CAD build for the part. Positions are in the model's coordinates, mm. Face numbers are marked on the shaded views. A direction names the side the tool comes from. Round coordinates to 2 decimals unless told otherwise and drop trailing zeros. Loops run counter-clockwise (first coordinate to the right, second up) from the corner with the lowest first, then second, coordinate; pieces in that order, holes last. Notation, with made-up numbers: M 78,47 L 114,47 A13 cw 114,67 Z; hole C -34.5,27.25 d6. An arc over 180 degrees is marked long. Put each result on its own line as item: value. Start each with the question number.
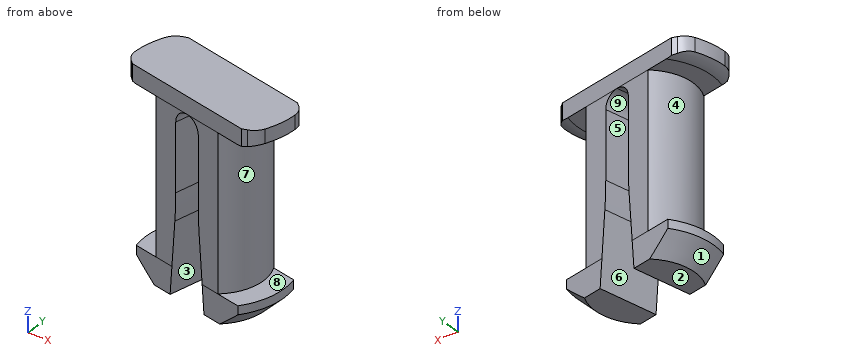
from build123d import *

# Parameters (mm, degrees)
BOSS_EXTRUDE1_DEPTH     = 1
CHAMFER1_SIZE           = 0.5
FILLET1_R               = 1
BOSS_EXTRUDE2_DEPTH     = 8.9
BOSS_EXTRUDE3_DEPTH     = 1.6
CUT_EXTRUDE1_DEPTH      = 63.654658492
CUT_EXTRUDE1_DEPTH_BACK = 63.654658492
FILLET2_R               = 20
FILLET3_R               = 0.8


# Some blends are built 0.0001 mm under size
with BuildPart() as part:
    # Sketch3 → Boss-Extrude1 (new body)
    with BuildSketch(Plane.XY.offset(7.5)):
        with BuildLine():
            Line((-59.471397705, 15.416079883), (-50.967479146, 13.468422533))
            ThreePointArc((-50.967479146, 13.468422533), (-51.028748516, 11.687143573), (-51.748854552, 10.056758353))
            Line((-51.748854552, 10.056758353), (-60.252773111, 12.004415704))
            ThreePointArc((-60.252773111, 12.004415704), (-60.191503741, 13.785694664), (-59.471397705, 15.416079883))
        make_face()
    extrude(amount=-BOSS_EXTRUDE1_DEPTH)

    # Chamfer1
    # the kernel refuses this chamfer: 0.5, 0.404802776 mm, written as the material it takes off along each edge
    with BuildSketch(Plane(origin=(-59.471397705, 15.416079883, 8.793542877), x_dir=(0.9747611941912204, -0.2232501160109568, 0), z_dir=(0, 0, -1))) as chamfer1_piece_1:
        with BuildLine():
            Line((CHAMFER1_SIZE, 0), (-0.128607842, 0.362926907))
            ThreePointArc((-0.128607842, 0.362926907), (-0.070555149, 0.18731274), (0, 0))
            Line((0, 0), (CHAMFER1_SIZE, 0))
        make_face()
    extrude(amount=3.587085755, mode=Mode.SUBTRACT)
    with BuildSketch(Plane(origin=(-50.967479146, 13.468422533, 8.793542877), x_dir=(-0.9747611941912215, 0.22325011601095288, 0), z_dir=(0, 0, -1)), Plane(origin=(-60.252773111, 12.004415704, 8.793542877), x_dir=(0.9747611941912214, -0.22325011601095318, 0), z_dir=(0, 0, -1))) as chamfer1_piece_2:
        with BuildLine():
            Line((CHAMFER1_SIZE, 0), (-0.128607842, -0.362926907))
            ThreePointArc((-0.128607842, -0.362926907), (-0.070555149, -0.18731274), (0, 0))
            Line((0, 0), (CHAMFER1_SIZE, 0))
        make_face()
    extrude(amount=3.587085755, mode=Mode.SUBTRACT)
    with BuildSketch(Plane(origin=(-51.748854552, 10.056758353, 8.793542877), x_dir=(0.5360100963407745, 0.8442115710061985, 0), z_dir=(0, 0, -1))) as chamfer1_piece_3:
        with BuildLine():
            Line((0.385040149, 0), (-CHAMFER1_SIZE * 0.334011510443, -CHAMFER1_SIZE * 0.942568995295))
            Line((-CHAMFER1_SIZE * 0.334011510443, -CHAMFER1_SIZE * 0.942568995295), (0, 0))
            ThreePointArc((0, 0), (0.200121413, 0.003938485), (0.385040149, 0))
        make_face()
    extrude(amount=3.587085755, mode=Mode.SUBTRACT)

    # Fillet1
    fillet1_edges = [part.edges().sort_by_distance(p)[0] for p in [
        (-50.923140687, 13.085943752, 7),
        (-51.542469145, 10.381813703, 7),
        (-59.677783112, 15.091024534, 7),
        (-60.29711157, 12.386894484, 7),
    ]]
    fillet(fillet1_edges, radius=FILLET1_R)

    # Sketch5 → Cut-Revolve1 (revolve, cut)
    with BuildSketch(Plane(origin=(0, 0, 0), x_dir=(0.9747611941912216, -0.22325011601095204, 0), z_dir=(0.22325011601095204, 0.9747611941912216, 0))):
        with BuildLine():
            Line((-60.95, -6.5), (-61.75, -6.5))
            Line((-61.75, -6.5), (-61.75, -6.7))
            ThreePointArc((-61.75, -6.7), (-61.362310563, -6.55075775), (-60.95, -6.5))
        make_face()
    revolve(axis=Axis((-55.610126129, 12.736419118, 6.5), (0, 0, 1)), mode=Mode.SUBTRACT)

    # Sketch6 → Boss-Extrude2 (add)
    with BuildSketch(Plane(origin=(0, 0, 6.5), x_dir=(-1, 0, 0), z_dir=(0, 0, -1))):
        with BuildLine():
            Line((58.131397429, 11.518555813), (56.780622787, 11.209187121))
            Line((56.780622787, 11.209187121), (55.999247381, 14.620851301))
            Line((55.999247381, 14.620851301), (57.350022023, 14.930219993))
            ThreePointArc((57.350022023, 14.930219993), (58.339457472, 13.361519443), (58.131397429, 11.518555813))
        make_face()
        with BuildLine():
            Line((55.221004876, 10.851986936), (53.870230234, 10.542618244))
            ThreePointArc((53.870230234, 10.542618244), (52.880794785, 12.111318794), (53.088854828, 13.954282424))
            Line((53.088854828, 13.954282424), (54.43962947, 14.263651115))
            Line((54.43962947, 14.263651115), (55.221004876, 10.851986936))
        make_face()
    extrude(amount=BOSS_EXTRUDE2_DEPTH)

    # Sketch7 → Boss-Extrude3 (add)
    with BuildSketch(Plane(origin=(0, 0, -2.4), x_dir=(-1, 0, 0), z_dir=(0, 0, -1))):
        with BuildLine():
            Line((54.43962947, 14.263651115), (51.713345578, 13.63924875))
            ThreePointArc((51.713345578, 13.63924875), (51.711081352, 11.843418654), (52.494720985, 10.227584571))
            Line((52.494720985, 10.227584571), (55.221004876, 10.851986936))
            Line((55.221004876, 10.851986936), (54.43962947, 14.263651115))
        make_face()
        with BuildLine():
            Line((55.999247381, 14.620851301), (58.725531273, 15.245253666))
            ThreePointArc((58.725531273, 15.245253666), (59.509170905, 13.629419582), (59.506906679, 11.833589487))
            Line((59.506906679, 11.833589487), (56.780622787, 11.209187121))
            Line((56.780622787, 11.209187121), (55.999247381, 14.620851301))
        make_face()
    extrude(amount=BOSS_EXTRUDE3_DEPTH)

    # Sketch8 → Cut-Revolve2 (revolve, cut)
    with BuildSketch(Plane(origin=(0, 0, 0), x_dir=(0.9747611941912216, -0.22325011601095204, 0), z_dir=(0.22325011601095204, 0.9747611941912216, 0))):
        Polygon((-61.05, 2.9), (-59.95, 4), (-61.05, 4), align=None)
    revolve(axis=Axis((-55.610126129, 12.736419118, 6.5), (0, 0, 1)), mode=Mode.SUBTRACT)

    # Sketch9 → Cut-Extrude1 (cut, two sides: drawn at the far end of the back side and taken through both)
    with BuildSketch(Plane(origin=(0.390687703, 1.70583209, 0), x_dir=(0.9747611941912216, -0.22325011601095204, 0), z_dir=(0.22325011601095204, 0.9747611941912216, 0)).offset(-CUT_EXTRUDE1_DEPTH_BACK)):
        Polygon((-58.25, 4), (-57.85, -1), (-57.85, 4), align=None)
        Polygon((-55.85, 4), (-56.25, -1), (-56.25, 4), align=None)
    extrude(amount=CUT_EXTRUDE1_DEPTH + CUT_EXTRUDE1_DEPTH_BACK, mode=Mode.SUBTRACT)

    # Fillet2
    # the kernel refuses this fillet: 20 mm, written as the material it takes off along each edge
    with BuildSketch(Plane(origin=(-53.993841362, 16.21006421, 1), x_dir=(0, 0, 1), z_dir=(-0.22325011601095204, -0.9747611941912216, 0))) as fillet2_piece_1:
        with BuildLine():
            CenterArc((FILLET2_R * 0.0399362039845, -FILLET2_R), FILLET2_R, 90, 4.57392126)
            Line((-FILLET2_R * 0.0398090182984, -FILLET2_R * 0.00318472146388), (0, 0))
            Line((0, 0), (FILLET2_R * 0.0399362039845, 0))
        make_face()
    extrude(amount=7.493620398, mode=Mode.SUBTRACT)
    with BuildSketch(Plane(origin=(-57.226410896, 9.262774027, 1), x_dir=(-0.07773254810353018, 0.01780313012597799, -0.9968152785361237), z_dir=(0.223250116010952, 0.9747611941912216, 0))) as fillet2_piece_2:
        with BuildLine():
            CenterArc((FILLET2_R * 0.0399362039845, FILLET2_R), FILLET2_R, 265.42607874, 4.57392126)
            Line((-FILLET2_R * 0.0398090182984, FILLET2_R * 0.00318472146388), (0, 0))
            Line((0, 0), (FILLET2_R * 0.0399362039845, 0))
        make_face()
    extrude(amount=7.493620398, mode=Mode.SUBTRACT)

    # Fillet3
    fillet3_edges = [part.edges().sort_by_distance(p)[0] for p in [
        (-54.830317173, 12.557819026, 6.5),
        (-56.389935084, 12.915019211, 6.5),
    ]]
    fillet(fillet3_edges, radius=FILLET3_R - 0.0001)  # a hair under: the kernel refuses the full size


solid = part.part
(1) Flat gauge pins, fed straight in: pin 1 Ø3 at (y, z) = (14, 4) entering from -X; pin 2 Ø5 at (x, z) = (-59, -2.5) entering from -Y; pin 3 Ø4 at (x, z) = (-56, 2.5) entering from -Y. Where does each tip first touch, or does it go through?
(2) Mould opens along X. For the marked faces 6, 7, 8 and 9 say: +X half, -X half, draft (parallel to the pull), parting line (faces both ways), or undercut.
(3) Cut at A-A on z = 3.5. List the corners of the cut face in (x, y).
(4) Drill centre lines: line 1 along Z through (x, y) = (-58.5, 14.85); line 2 along Z through (x, y) = (-52.5, 13.5); line 3 along X through (y, z) = (12.1, 5.75) (3 decimals). Where is each one in solid material? Low to high.
(5) Tool access for the marked faces 1, 2, 3, 4 and 5: list every direction of +Z, -Z, +X, -X, +Y, -Y with a clear straight run to the whole face (end or side of a thin tool).
(6) Cut at B-B on z = 6. List the corners of the cut face in (x, y), and give its area (3 significant figures).
Taken from the geometry:
1. pin 1: x = -58.41
1. pin 2: y = 11.25
1. pin 3: y = 10.57
2. face 6: undercut
2. face 7: +X half
2. face 8: draft
2. face 9: undercut
3. outline: M -58.13,11.52 L -56.78,11.21 L -56,14.62 L -57.35,14.93 A2.8 ccw Z; M -55.22,10.85 L -53.87,10.54 A2.8 ccw -53.09,13.95 L -54.44,14.26 Z
4. line 1: -3.32 to -2.4, 6.5 to 7.5
4. line 2: -3.7 to -2.4, 6.5 to 7.5
4. line 3: -58.337 to -56.575, -54.937 to -52.883
5. face 1: -Z, -X
5. face 2: -Z, +X, -X, +Y, -Y
5. face 3: -Z, -Y
5. face 4: -X
5. face 5: -Z, +Y
6. outline: M -58.13,11.52 L -56.72,11.2 L -55.94,14.61 L -57.35,14.93 A2.8 ccw Z; M -55.28,10.87 L -53.87,10.54 A2.8 ccw -53.09,13.95 L -54.5,14.28 Z
6. area: 13.0 mm2
